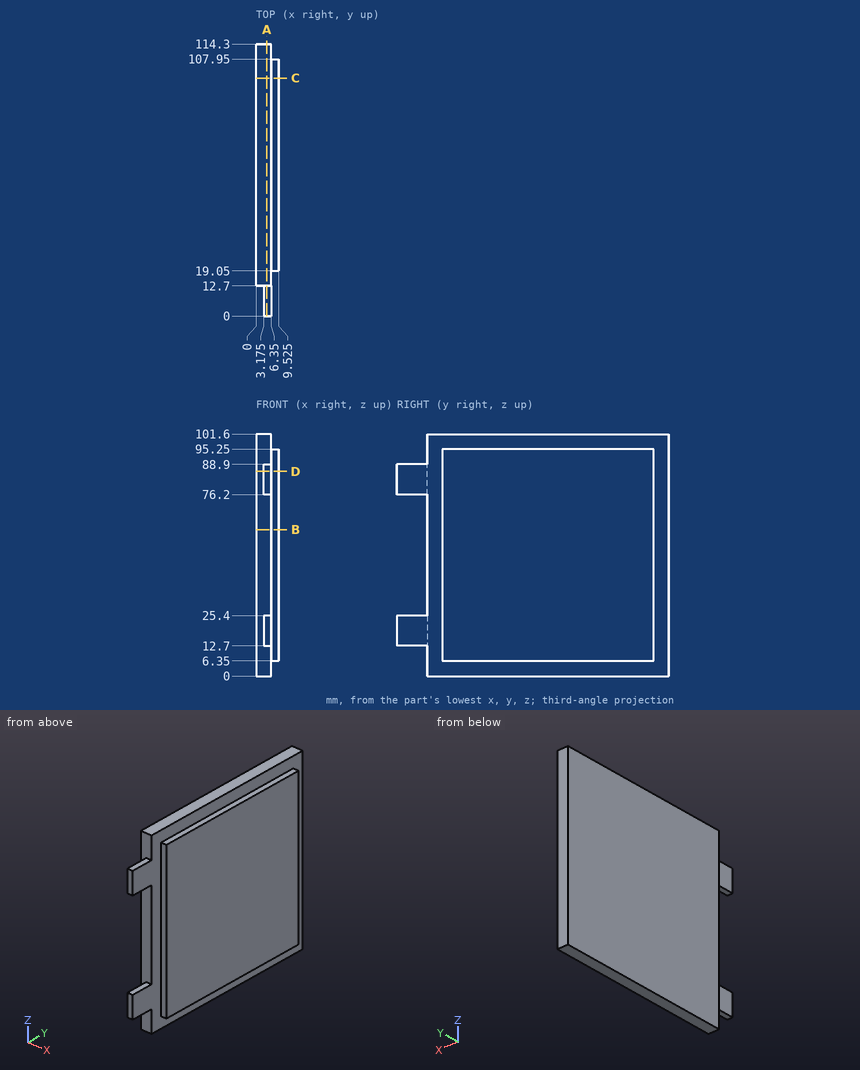
The figure shows three views and two pictorial views of one solid part (mm, origin at its lowest corner). Answer the questions. Round coordinates to 2 decimals unless told otherwise and drop trailing zeros. Loops run counter-clockwise (first coordinate to the right, second up) from the corner with the lowest first, then second, coordinate; pieces in that order, holes last. Notation, with made-up numbers: (46.25, -11) -> (81.25, -11) arc R29 ccw to (81.25, 22) -> close; hole circle Ø1 at (49.25, 86). An arc over 180 degrees is marked (long way). Use one line per item in the form item = value.
(1) Straight lines are drawn through the part: line 1 (Z direction, x = 4.5, y = 7.5); line 2 (Y direction, x = 3, z = 36); line 3 (Y direction, x = 8.5, z = 89). For each, find the intervals that lie inside material, in ascending order.
Answer list:
line_1 = 12.7 to 25.4, 76.2 to 88.9
line_2 = 12.7 to 114.3
line_3 = 19.05 to 107.95
(2) Find section B-B on z = 61.5. Give the vertices of the cut face in (x, y) (3 decimals), then the cut area to 3 significant figures.
Answer list:
outline = (0, 12.7) -> (6.35, 12.7) -> (6.35, 19.05) -> (9.525, 19.05) -> (9.525, 107.95) -> (6.35, 107.95) -> (6.35, 114.3) -> (0, 114.3) -> close
area = 927 mm2
(3) Flat-ended cylindrical pins translate along their axes: P1, Ø2.5, axis at x = 8.5, z = 54, coming from the -Y side; P2, Ø1.6, axis at x = 5.5, y = 4, coming from the +Z side; P3, Ø1, axis at x = 8, y = 55, coming from the +Z side. Find the tip coordinate at first contact, or state that the pin passes through.
Answer list:
P1 = 19.05
P2 = 88.9
P3 = 95.25
(4) Find section D-D on z = 86. Give the vertices of the cut face in (x, y) (3 decimals), then the cut area to 3 significant figures.
Answer list:
outline = (0, 12.7) -> (3.175, 12.7) -> (3.175, 0) -> (6.35, 0) -> (6.35, 19.05) -> (9.525, 19.05) -> (9.525, 107.95) -> (6.35, 107.95) -> (6.35, 114.3) -> (0, 114.3) -> close
area = 968 mm2
(5) Find section A-A on x = 4.5. Give the vertices of the cut face in (y, z), then the cut area to 3 significant figures.
Answer list:
outline = (0, 12.7) -> (12.7, 12.7) -> (12.7, 0) -> (114.3, 0) -> (114.3, 101.6) -> (12.7, 101.6) -> (12.7, 88.9) -> (0, 88.9) -> (0, 76.2) -> (12.7, 76.2) -> (12.7, 25.4) -> (0, 25.4) -> close
area = 10,600 mm2
(6) Find section C-C on y = 100. Give the vertices of the cut face in (x, z) (3 decimals).
Answer list:
outline = (0, 0) -> (6.35, 0) -> (6.35, 6.35) -> (9.525, 6.35) -> (9.525, 95.25) -> (6.35, 95.25) -> (6.35, 101.6) -> (0, 101.6) -> close
